Autodesk Inventor part; units mm, degrees
ref_plane "YZ Plane" through (0, 0, 0) normal (1, 0, 0) x (0, 1, 0)
ref_plane "XZ Plane" through (0, 0, 0) normal (0, 1, 0) x (-1, 0, 0)
ref_plane "XY Plane" through (0, 0, 0) normal (0, 0, 1) x (1, 0, 0)
sketch "Sketch2" plane through (0, 0, 0) normal (0, 1, 0) x (-1, 0, 0)
  line L0 (0, 0) -> (69.85, 0)
  line L1 (69.85, 0) -> (69.85, -25.4) construction
  line L2 (69.85, -25.4) -> (0, -25.4)
  line L3 (0, -25.4) -> (0, 0)
  arc A0 (69.85, -25.4) -> (69.85, 0) centre (69.85, -12.7) ccw
  dimension "d0" = 25.4
  dimension "d1" = 69.85
extrude "Extrusion1" add sketch "Sketch2" along normal blind 19.05
ref_plane "Work Plane1" through (0, 19.05, 0) normal (0.7071068, -0.7071068, 0) x (0, 0, -1)
mirror "Mirror1" about plane through (0, 19.05, 0) normal (0.7071068, -0.7071068, 0) of "Extrusion1"
sketch "Sketch3" plane through (-69.85, 19.05, 0) normal (0, 0, 1) x (1, 0, 0)
  line L0 (50.8, -69.85) -> (50.8, -19.05)
  line L1 (-50.8, -120.65) -> (50.8, -120.65)
  line L2 (50.8, -120.65) -> (50.8, -19.05)
  line L3 (50.8, -19.05) -> (-50.8, -19.05)
  line L4 (-50.8, -19.05) -> (-50.8, -120.65)
  line L5 (-50.8, -120.65) -> (50.8, -19.05) construction
  line L6 (50.8, -120.65) -> (-50.8, -19.05) construction
  point P0 (0, -69.85)
  point P1 (0, -69.85)
  dimension "d6" = 101.6
extrude "Extrusion2" add sketch "Sketch3" against normal up to surface (25.4 mm away)
hole "Hole1" at (-69.85, -50.8, 0) direction (0, 0, -1) diameter 76.2 end through all
sketch "Sketch4" plane through (0, 19.05, 0) normal (1, 0, 0) x (0, 0, -1)
  arc A0 (0, -69.85) -> (25.4, -69.85) centre (12.7, -69.85) ccw
  point P0 (0, -19.05)
hole "Hole2" at (0, -50.8, -12.7) direction (-1, 0, 0) diameter 12.7 end up to surface
sketch "Sketch5" plane through (0, 19.05, 0) normal (0, 1, 0) x (1, 0, 0)
  arc A0 (-69.85, 25.4) -> (-69.85, 0) centre (-69.85, 12.7) ccw
  point P0 (0, 0)
hole "Hole3" at (-69.85, 19.05, -12.7) direction (0, -1, 0) diameter 12.7 end up to surface
properties part number "PivotHolder"
The listing builds one solid part. Answer for the finished solid, in the listing's coordinates (mm). A direction names the side the tool comes from. Give positions to 0.01 mm unless a question says otherwise; leave off trailing zeros. Loops run counter-clockwise (first coordinate to the right, second up) from the corner with the lowest first, then second, coordinate; pieces in that order, holes last. Notation, with made-up numbers: M 18.25,2.5 L 45.25,2.5 A29 ccw 45.25,41.5 Z; hole C -9.75,5.25 d6. An arc over 180 degrees is marked long. One line per item, written item: value.
1. Find the intervals of material crossed by probe 1 along Z at (x, y) = (-69.85, -5.5); probe 2 along Y at (x, z) = (-12.5, -12.7); probe 3 along Y at (x, z) = (-69.85, -16.5), in increasing order.
Found:
probe 1: -25.4 to -19.05, -6.35 to 0
probe 2: -63.5 to -57.15, -44.45 to 19.05
probe 3: -101.6 to -88.9
2. Each of these flat-tipped pins is pushed along its axis until it touches: P1, Ø1.5, axis at x = -75.5, y = 1.5, coming from the -Z side; P2, Ø12.5, axis at y = -71.5, z = -10, coming from the +X side; P3, Ø7.5, axis at x = -102, z = -10, coming from the +Y side. Where does it stop, or does it pass through?
Found:
P1: z = -24.42
P2: x = -19.05
P3: y = 0
3. Section D-D on y = -31.5 is taken. Determine the outline of the cut face in (x, z), plus the area to 3 significant figures.
Found:
outline: M -120.65,-25.4 L -102.7,-25.4 L -102.7,0 L -120.65,0 Z; M -37,-25.4 L 0,-25.4 L 0,0 L -37,0 Z
area: 1,400 mm^2
4. Section B-B on y = 8 is taken. Determine the outline of the cut face in (x, z), plus the area to 3 significant figures.
Found:
outline: M -69.85,-25.4 L 0,-25.4 L 0,0 L -69.85,0 A12.7 ccw Z; hole C -69.85,-12.7 d12.7
area: 1,900 mm^2
5. Section A-A on z = -12.7 is taken. Determine the outline of the cut face in (x, y), plus the area to 3 significant figures.
Found:
outline: M -120.65,-101.6 L -19.05,-101.6 L -19.05,-63.5 L 0,-63.5 L 0,-57.15 L -32.28,-57.15 A38.1 cw long -76.2,-13.23 L -76.2,19.05 L -82.55,19.05 L -82.55,0 L -120.65,0 Z; M -63.5,-13.23 A38.1 cw -32.28,-44.45 L 0,-44.45 L 0,19.05 L -63.5,19.05 Z
area: 7,730 mm^2
6. Section C-C on x = -34 is taken. Determine the outline of the cut face in (y, z), plus the area to 3 significant figures.
Found:
outline: M -101.6,-25.4 L -63.7,-25.4 L -63.7,0 L -101.6,0 Z; M -37.9,-25.4 L 19.05,-25.4 L 19.05,0 L -37.9,0 Z
area: 2,410 mm^2
7. For faces 1 (the face through (-16.4, -57.1, -11.9)), 2 (the face through (-82.547, 9.392, -12.421)), 3 (the face through (-76.146, 2.683, -13.527)), 4 (the face through (-71, -101.6, -13)), determine the directions among +Z, -Z, +X, -X, +Y, -Y from which every point of the face is accessible in a straight line to the end or side of a thin tool.
Found:
face 1: +X
face 2: -X, +Y
face 3: +Y
face 4: +Z, -Z, +X, -X, -Y
8. For a pull along Y with two mould halves and no side action, classify faces 5 (the face through (-48, -14, 0)), 6 (the face through (-9.658, -63.497, -12.979)), 7 (the face through (-81.29, -87.14, -12.88)), 8 (the face through (-101, 0, -13)) as pulls with the +Y half, pulls with the -Y half, needs draft (parallel to the pull), parting line crosses it, or undercut.
Found:
face 5: needs draft
face 6: pulls with the -Y half
face 7: undercut
face 8: pulls with the +Y half
